Here's the drawing with two shaded views (mm, measured from the low corner). I have some questions. A direction names the side the tool comes from. Give positions to 0.01 mm unless a question says otherwise; leave off trailing zeros. Loops run counter-clockwise (first coordinate to the right, second up) from the corner with the lowest first, then second, coordinate; pieces in that order, holes last.
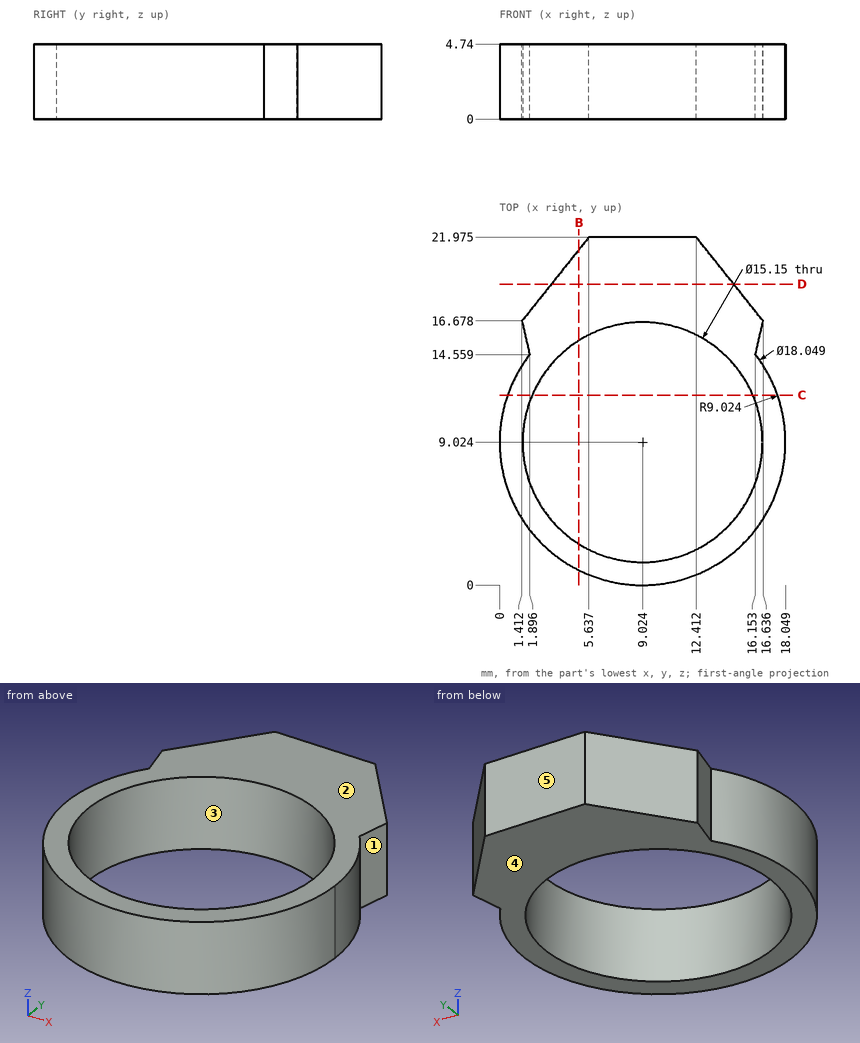
(1) Suppose I cut it at D-D on y = 19. List the corners of the cut face in (x, z) for me (1 decimal), plus the area to 3 significant figures.
Returned:
outline: (3.3, 0) - (14.8, 0) - (14.8, 4.7) - (3.3, 4.7) - close
area: 54.6 mm2
(2) Suppose I cut it at B-B on x = 5. List the corners of the cut face in (y, z) for me.
Returned:
outline: (0.95, 0) - (2.61, 0) - (2.61, 4.74) - (0.95, 4.74) - close; (15.44, 0) - (21.18, 0) - (21.18, 4.74) - (15.44, 4.74) - close
(3) Please list where these lines run through material, in increasing order: probe 1 along X at (y, z) = (3.25, 0.55) (1 decimal); probe 2 along X at (y, z) = (6.25, 0.85) (1 decimal); probe 3 along Y at (x, z) = (14.25, 0.35) (1 decimal).
Returned:
probe 1: x = 2.1 to 4.1, 13.9 to 16
probe 2: x = 0.4 to 2, 16.1 to 17.6
probe 3: y = 1.7 to 3.5, 14.5 to 19.7
(4) Will this pin go through, and if not, where does the flat tip stop? P1, Ø1, axis at x = 5.5, z = 1, coming from the -Y side.
Returned:
P1: stops at y = 0.52
(5) Thinking about a two-plate mould opening in Y: for the marked faces 3, 4 and 5, which applies, pulls with the +Y half, pulls with the -Y half, needs draft (parallel to the pull), parting line crosses it, or undercut?
Returned:
face 3: undercut
face 4: needs draft
face 5: pulls with the +Y half
(6) Which directions (+Z, -Z, +X, -X, +Y, -Y) give clear straight access to the entire face, cutting with the end or side of a thin tool? Please do the marked faces 1 and 2.
Returned:
face 1: +Z, -Z, +X
face 2: +Z, +X, -X, +Y, -Y
(7) Suppose I cut it at C-C on y = 12. List the corners of the cut face in (x, z) for me (1 decimal).
Returned:
outline: (0.5, 0) - (2.1, 0) - (2.1, 4.7) - (0.5, 4.7) - close; (16, 0) - (17.5, 0) - (17.5, 4.7) - (16, 4.7) - close
